Can you work these out from the model? Positions are in its coordinate system, mm. Round coordinates to 2 decimals unless told otherwise and drop trailing zeros. Order: outer loops, then holes, each group sorted by start corner. A loop starts at its lowest first (then second) coordinate and runs counter-clockwise, first axis right, second up. Notation, with made-up numbers: (7.25, 53.5) - (58.25, 53.5) arc R13 ccw to (58.25, 68.5) - close; hole circle Ø2 at (51.5, 47). An arc over 180 degrees is marked (long way). Write item = value, one per line.
from build123d import *

# Parameters (mm, degrees)
SKETCH1_W           = 50
SKETCH1_H           = 30
BOSS_EXTRUDE1_DEPTH = 1.6
SKETCH2_W           = 10
SKETCH2_H           = 1.6
BOSS_EXTRUDE2_DEPTH = 1.6
CUT_EXTRUDE1_DEPTH  = 60.170262802
FILLET1_R           = 1


with BuildPart() as part:
    # Sketch1 → Boss-Extrude1 (new body)
    with BuildSketch(Plane.XY):
        with Locations((25, 15)):
            Rectangle(SKETCH1_W, SKETCH1_H)
    extrude(amount=BOSS_EXTRUDE1_DEPTH)

    # Sketch2 → Boss-Extrude2 (add)
    with BuildSketch(Plane.XY.offset(1.6)):
        with Locations((5, 30.8)):
            Rectangle(SKETCH2_W, SKETCH2_H)
        with Locations((45, 30.8)):
            Rectangle(SKETCH2_W, SKETCH2_H)
        with Locations((45, -0.8)):
            Rectangle(SKETCH2_W, SKETCH2_H)
        with Locations((5, -0.8)):
            Rectangle(SKETCH2_W, SKETCH2_H)
    extrude(amount=-BOSS_EXTRUDE2_DEPTH)

    # Sketch3 → Cut-Extrude1 (cut, through all)
    with BuildSketch(Plane.XY.offset(1.6)):
        Polygon((4, 26), (4, 4), (23, 15), align=None)
        Polygon((9.454545455, 26), (40.545454545, 26), (25, 17), align=None)
        Polygon((25, 13), (9.454545455, 4), (40.545454545, 4), align=None)
        Polygon((27, 15), (46, 26), (46, 4), align=None)
    extrude(amount=-CUT_EXTRUDE1_DEPTH, mode=Mode.SUBTRACT)

    # Fillet1
    fillet1_edges = [part.edges().sort_by_distance(p)[0] for p in [
        (46, 4, 0.8),
        (27, 15, 0.8),
        (46, 26, 0.8),
        (25, 17, 0.8),
        (9.454545455, 26, 0.8),
        (40.545454545, 26, 0.8),
        (25, 13, 0.8),
        (40.545454545, 4, 0.8),
        (9.454545455, 4, 0.8),
        (4, 26, 0.8),
        (23, 15, 0.8),
        (4, 4, 0.8),
    ]]
    fillet(fillet1_edges, radius=FILLET1_R)


solid = part.part
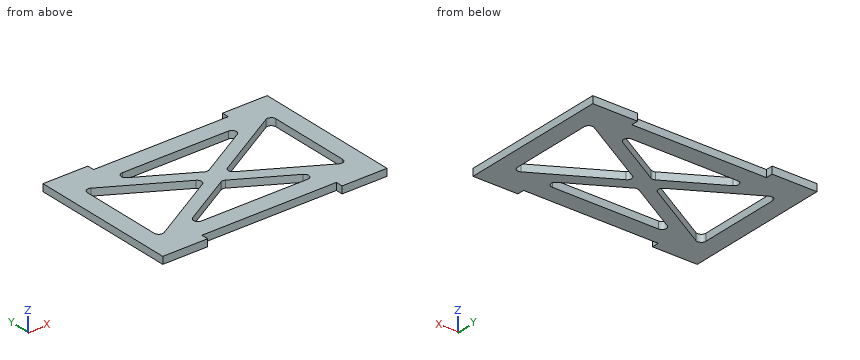
(1) If we section it at D-D (x = 24): Write out the boundary of the cut face in (y, z).
Computed:
outline = (0, 0) - (4, 0) - (4, 1.6) - (0, 1.6) - close; (12.42, 0) - (17.58, 0) - (17.58, 1.6) - (12.42, 1.6) - close; (26, 0) - (30, 0) - (30, 1.6) - (26, 1.6) - close
(2) Will this pin go through, and if not, where does the flat tip stop? P1, Ø0.5, axis at x = 25.5, z = 0.5, coming from the -Y side.
Computed:
P1 = 0
(3) If I drill on line 1 (Y direction, x = 16.5, z = 0.25); line 2 (X direction, y = 17.5, z = 1.4); line 3 (X direction, y = 23, z = 1.15), over which ranges is the centre line in solid material (lowest first)? Write a range as from..to.
Computed:
line_1 = 0..4, 8.08..11.24, 18.76..21.92, 26..30
line_2 = 0..4, 18.68..24.14, 25.86..31.32, 46..50
line_3 = 0..4, 9.18..14.64, 35.36..40.82, 46..50
(4) If we section it at A-A (x = 45.5): Write out the boundary of the cut face in (y, z), plus the area to 3 significant figures.
Computed:
outline = (-1.6, 0) - (4.87, 0) - (4.87, 1.6) - (-1.6, 1.6) - close; (25.13, 0) - (31.6, 0) - (31.6, 1.6) - (25.13, 1.6) - close
area = 20.7 mm^2
(5) If we section it at C-C (x = 35.5): Write out the boundary of the cut face in (y, z), plus the area to 3 significant figures.
Computed:
outline = (0, 0) - (4, 0) - (4, 1.6) - (0, 1.6) - close; (6.92, 0) - (10.08, 0) - (10.08, 1.6) - (6.92, 1.6) - close; (19.92, 0) - (23.08, 0) - (23.08, 1.6) - (19.92, 1.6) - close; (26, 0) - (30, 0) - (30, 1.6) - (26, 1.6) - close
area = 22.9 mm^2
(6) If we section it at B-B (y = 18): Write out the boundary of the cut face in (x, z), plus the area to 3 significant figures.
Computed:
outline = (0, 0) - (4, 0) - (4, 1.6) - (0, 1.6) - close; (17.82, 0) - (23.27, 0) - (23.27, 1.6) - (17.82, 1.6) - close; (26.73, 0) - (32.18, 0) - (32.18, 1.6) - (26.73, 1.6) - close; (46, 0) - (50, 0) - (50, 1.6) - (46, 1.6) - close
area = 30.3 mm^2
